```python
from build123d import *

# Parameters (mm, degrees)
F1_DEPTH = 100
F2_SIZE  = 2.99999
F3_SIZE  = 1
F4_R     = 6
F5_DEPTH = 10
F6_SIZE  = 1


# Not quite as in the source:
# - a fillet or chamfer is up to 0.001 mm smaller than in the source, because OpenCascade refuses the exact size


with BuildPart() as f1:
    # F0 (on Right) → F1 (new body)
    with BuildSketch(Plane.YZ):
        with BuildLine():
            Line((45, 36.1919924617), (0, 36.1919924617))
            Line((0, 36.1919924617), (0, 26.1919924617))
            Line((0, 26.1919924617), (41, 26.1919924617))
            ThreePointArc((41, 26.1919924617), (43.8284271247, 25.0204195864), (45, 22.1919924617))
            Line((45, 22.1919924617), (45, 8.2077106759))
            ThreePointArc((45, 8.2077106759), (47.9289321881, 1.136642864), (55, -1.7922893241))
            Line((55, -1.7922893241), (90, -1.7922893241))
            Line((90, -1.7922893241), (90, 5.2077106759))
            ThreePointArc((90, 5.2077106759), (89.1213203436, 7.3290310195), (87, 8.2077106759))
            Line((87, 8.2077106759), (59, 8.2077106759))
            ThreePointArc((59, 8.2077106759), (56.1715728753, 9.3792835511), (55, 12.2077106759))
            Line((55, 12.2077106759), (55, 26.1919924617))
            ThreePointArc((55, 26.1919924617), (52.0710678119, 33.2630602735), (45, 36.1919924617))
        make_face()
        with BuildLine():
            Line((0, 26.1919924617), (0, 36.1919924617))
            Line((0, 36.1919924617), (-45, 36.1919924617))
            ThreePointArc((-45, 36.1919924617), (-52.0710678119, 33.2630602735), (-55, 26.1919924617))
            Line((-55, 26.1919924617), (-55, 12.2077106759))
            ThreePointArc((-55, 12.2077106759), (-56.1715728753, 9.3792835511), (-59, 8.2077106759))
            Line((-59, 8.2077106759), (-87, 8.2077106759))
            ThreePointArc((-87, 8.2077106759), (-89.1213203436, 7.3290310195), (-90, 5.2077106759))
            Line((-90, 5.2077106759), (-90, -1.7922893241))
            Line((-90, -1.7922893241), (-55, -1.7922893241))
            ThreePointArc((-55, -1.7922893241), (-47.9289321881, 1.136642864), (-45, 8.2077106759))
            Line((-45, 8.2077106759), (-45, 22.1919924617))
            ThreePointArc((-45, 22.1919924617), (-43.8284271247, 25.0204195864), (-41, 26.1919924617))
            Line((-41, 26.1919924617), (0, 26.1919924617))
        make_face()
    extrude(amount=F1_DEPTH)

    # F2 (size 3 in the source; OpenCascade refuses exactly that, so slightly less here)
    f2_edges = [f1.edges().sort_by_distance(p)[0] for p in [
        (0, -90, 1.707711),
        (0, -89.12132, 7.329031),
        (0, -73, 8.207711),
        (0, -56.171573, 9.379284),
        (0, -55, 19.199852),
        (0, -52.071068, 33.26306),
        (0, 0, 36.191992),
        (0, 52.071068, 33.26306),
        (100, 0, 36.191992),
    ]]
    chamfer(f2_edges, length=F2_SIZE)

    # F3
    f3_edges = [f1.edges().sort_by_distance(p)[0] for p in [
        (100, 0, 26.191992),
        (0, 0, 26.191992),
    ]]
    chamfer(f3_edges, length=F3_SIZE)

    # F4 (on face) → F5 (cut)
    with BuildSketch(Plane.XY.offset(36.1919924617)):
        with Locations((18, -30)):
            Circle(F4_R)
        with Locations((82, -30)):
            Circle(F4_R)
        with Locations((82, 30)):
            Circle(F4_R)
        with Locations((18, 30)):
            Circle(F4_R)
    extrude(amount=-F5_DEPTH, mode=Mode.SUBTRACT)

    # F6
    f6_edges = [f1.edges().sort_by_distance(p)[0] for p in [
        (12, 30, 36.191992),
        (76, 30, 36.191992),
        (88, -30, 31.191992),
        (76, -30, 36.191992),
        (76, -30, 26.191992),
        (12, -30, 36.191992),
        (76, 30, 26.191992),
        (12, 30, 26.191992),
        (12, -30, 26.191992),
    ]]
    chamfer(f6_edges, length=F6_SIZE)


solid = f1.part
```
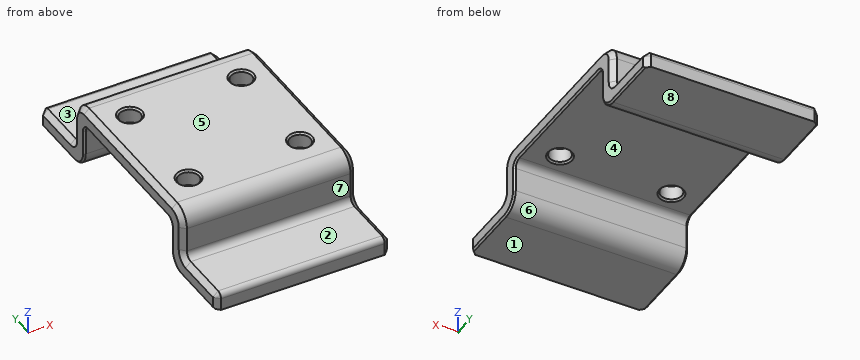
Check sheet for the modelled part. Datum: model origin and axes. Units: mm. Face numbers are marked on the shaded views. A direction names the side the tool comes from. Round coordinates to 2 decimals unless told otherwise and drop trailing zeros. Order: outer loops, then holes, each group sorted by start corner. A loop starts at its lowest first (then second) coordinate and runs counter-clockwise, first axis right, second up. Notation, with made-up numbers: (24.5, 87.25) - (41.5, 87.25) arc R27 ccw to (41.5, 119.25) - close; hole circle Ø11 at (49.5, 32). An arc over 180 degrees is marked (long way). Answer as CSV lines item,"result". Start each with the question number.
1) Draft check along Y on the marked faces 6, 7 and 8. Enter one of: +Y half, -Y half, draft (parallel to the pull), parting line (faces both ways), or undercut.
2) Depth check by flat-ended pin: pin 1 (10 mm diameter, centred on y = 65.5, z = 13.5, fed in from +X); pin 2 (15.5 mm diameter, centred on x = 68, z = 16.5, fed in from +Y); pin 3 (8.5 mm diameter, centred on x = 47, y = 66.5, fed in from +Z); pin 4 (1 mm diameter, centred on x = 58.5, y = -36.5, fed in from -Z). Enter the tip coordinate at first touch or a pass-through.
3) Tool access check on the marked faces 1, 2, 3, 4 and 5. Record the directions out of +Z, -Z, +X, -X, +Y, -Y that give a thin tool (end or side, any length) a straight path to the whole face; none if there is none.
4) Section check A-A (z = 14.5). Record the cut outline in (x, y), then the cut area to 3 significant figures.
5) Section check B-B (y = 30). Record the cut outline in (x, z), then the cut area to 3 significant figures.
6) Scan lines: probe 1 along Y at (x, z) = (95, 20); probe 2 along Y at (x, z) = (18, 32); probe 3 along Y at (x, z) = (82, 30). Record each from-to range of solid material in increasing order.
7) Section check C-C (x = 40.5). Record the cut outline in (y, z), then the cut area to 3 significant figures.
Determined:
1,face 6,"undercut"
1,face 7,"-Y half"
1,face 8,"draft"
2,pin 1,"through"
2,pin 2,"y = 56.99"
2,pin 3,"z = 8.21"
2,pin 4,"z = 26.19"
3,face 1,"-Z, +X, -X, +Y, -Y"
3,face 2,"+Z, +X, -X, -Y"
3,face 3,"+Z, +X, -X, +Y"
3,face 4,"-Z, +X, -X"
3,face 5,"+Z, +X, -X, +Y, -Y"
4,outline,"(0, -52) - (3, -55) - (97, -55) - (100, -52) - (100, -46) - (99, -45) - (1, -45) - (0, -46) - close; (0, 46) - (1, 45) - (99, 45) - (100, 46) - (100, 52) - (97, 55) - (3, 55) - (0, 52) - close"
4,area,"1,980 mm^2"
5,outline,"(0, 27.19) - (1, 26.19) - (11, 26.19) - (12, 27.19) - (12, 35.19) - (11, 36.19) - (3, 36.19) - (0, 33.19) - close; (24, 27.19) - (25, 26.19) - (75, 26.19) - (76, 27.19) - (76, 35.19) - (75, 36.19) - (25, 36.19) - (24, 35.19) - close; (88, 27.19) - (89, 26.19) - (99, 26.19) - (100, 27.19) - (100, 33.19) - (97, 36.19) - (89, 36.19) - (88, 35.19) - close"
5,area,"746 mm^2"
6,probe 1,"-55 to -45, 45 to 55"
6,probe 2,"-53.14 to -36, -24 to 24, 36 to 53.14"
6,probe 3,"-54.25 to -36, -24 to 24, 36 to 54.25"
7,outline,"(-90, -1.79) - (-55, -1.79) arc R10 ccw to (-45, 8.21) - (-45, 22.19) arc R4 cw to (-41, 26.19) - (41, 26.19) arc R4 cw to (45, 22.19) - (45, 8.21) arc R10 ccw to (55, -1.79) - (90, -1.79) - (90, 5.21) arc R3 ccw to (87, 8.21) - (59, 8.21) arc R4 cw to (55, 12.21) - (55, 26.19) arc R10 ccw to (45, 36.19) - (-45, 36.19) arc R10 ccw to (-55, 26.19) - (-55, 12.21) arc R4 cw to (-59, 8.21) - (-87, 8.21) arc R3 ccw to (-90, 5.21) - close"
7,area,"2,280 mm^2"
